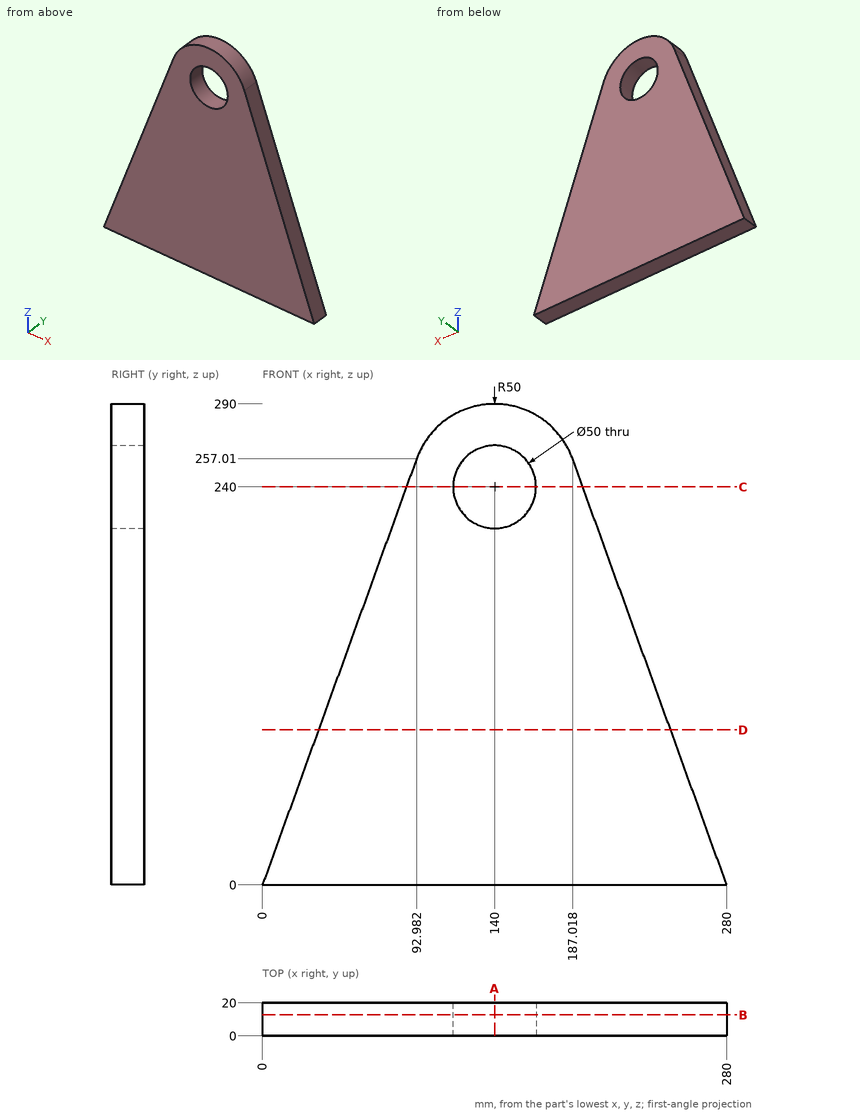
Could you check a few things on this drawing? It's one solid part, dimensions in mm from its lowest x, y, z. Give positions to 0.01 mm unless a question says otherwise; leave off trailing zeros. Order: outer loops, then holes, each group sorted by start corner. A loop starts at its lowest first (then second) coordinate and runs counter-clockwise, first axis right, second up. Notation, with made-up numbers: (-2, 79) - (9, 79) arc R20 cw to (9, 109) - close; hole circle Ø8 at (79.25, 69). An arc over 180 degrees is marked (long way). Answer as a JSON object with one key per item and string values. Group by question number.
Item 1: Please list where these lines run through material, in increasing order: probe 1 along X at (y, z) = (5.5, 230.5) (1 decimal); probe 2 along Z at (x, y) = (148, 16.5) (1 decimal); probe 3 along X at (y, z) = (7, 254.5) (1 decimal).
Item 2: If we section it at A-A on x = 140: Please give me the cut outline in (y, z), and give its area (3 significant figures).
Item 3: For P1, Ø5, axis at y = 13, z = 179.5, coming from the +X side (1 decimal); P2, Ø10, axis at y = 8, z = 244, coming from the +X side; P3, Ø6, axis at y = 5, z = 167, coming from the +X side, each with a flat end and sliding along its axis, tell me the tip position at first contact or that it passes through.
Item 4: If we section it at B-B on y = 12.75: Please give me the cut outline in (x, z), and give its area (3 significant figures).
Item 5: If we section it at C-C on z = 240: Please give me the cut outline in (x, y), and give its area (3 significant figures).
Item 6: If we section it at D-D on z = 93.5: Please give me the cut outline in (x, y), and give its area (3 significant figures).
Result set:
{
 "1": {"probe 1": "83.4 to 116.9, 163.1 to 196.6", "probe 2": "0 to 216.3, 263.7 to 289.4", "probe 3": "92.1 to 119.6, 160.4 to 187.9"},
 "2": {"outline": "(0, 0) - (20, 0) - (20, 215) - (0, 215) - close; (0, 265) - (20, 265) - (20, 290) - (0, 290) - close", "area": "4,800 mm²"},
 "3": {"P1": "x = 216", "P2": "x = 193.53", "P3": "x = 220.67"},
 "4": {"outline": "(0, 0) - (280, 0) - (187.02, 257.01) arc R50 ccw to (92.98, 257.01) - close; hole circle Ø50 at (140, 240)", "area": "48,400 mm²"},
 "5": {"outline": "(86.83, 0) - (115, 0) - (115, 20) - (86.83, 20) - close; (165, 0) - (193.17, 0) - (193.17, 20) - (165, 20) - close", "area": "1,130 mm²"},
 "6": {"outline": "(33.83, 0) - (246.17, 0) - (246.17, 20) - (33.83, 20) - close", "area": "4,250 mm²"}
}
